The listing builds one solid part. Answer for the finished solid, in the listing's coordinates (mm). Face numbers are marked on the shaded views. A direction names the side the tool comes from. Coordinates: 2 decimals unless noted, no trailing zeros. Order: outer loops, then holes, each group sorted by start corner. A loop starts at its lowest first (then second) coordinate and runs counter-clockwise, first axis right, second up. Notation, with made-up numbers: (78, 56.25) -> (91, 56.25) arc R23 ccw to (91, 82.25) -> close; hole circle Ø1 at (88, 30). An arc over 180 degrees is marked (long way). Answer in a Markdown table with one row per item.
```python
from build123d import *

# Parameters (mm, degrees)
BOSS_EXTRU_1_DEPTH      = 17
ESQUISSE2_W             = 26
ESQUISSE2_H             = 16
BOSS_EXTRU_2_DEPTH      = 44
ENL_V_MAT_EXTRU_1_DEPTH = 12
ESQUISSE4_W             = 35
ESQUISSE4_H             = 16.981352254
BOSS_EXTRU_3_DEPTH      = 16
ESQUISSE5_W             = 35
ESQUISSE5_H             = 10
BOSS_EXTRU_4_DEPTH      = 44
ESQUISSE6_W             = 36.437850792
ESQUISSE6_H             = 10
BOSS_EXTRU_5_DEPTH      = 10
CONG_1_SIZE             = 10
CONG_1_SIZE_2           = 8
ESQUISSE8_R             = 5
ENL_V_MAT_EXTRU_2_DEPTH = 10


with BuildPart() as part:
    # Esquisse1 → Boss.-Extru.1 (new body)
    with BuildSketch(Plane.XY):
        Polygon((0, 0), (94, 0), (94, 9), (79, 16), (15, 16), (0, 9), align=None)
    extrude(amount=-BOSS_EXTRU_1_DEPTH)

    # Esquisse2 → Boss.-Extru.2 (add)
    with BuildSketch(Plane.XY):
        with Locations((47, 8)):
            Rectangle(ESQUISSE2_W, ESQUISSE2_H)
    extrude(amount=BOSS_EXTRU_2_DEPTH)

    # Esquisse3 → Enlèv. mat.-Extru.1 (cut)
    with BuildSketch(Plane(origin=(0, 16, 0), x_dir=(1, 0, 0), z_dir=(0, 1, 0))):
        with BuildLine():
            Line((38, -44), (56, -44))
            Line((56, -44), (56, -19))
            ThreePointArc((56, -19), (47, -10), (38, -19))
            Line((38, -19), (38, -44))
        make_face()
    extrude(amount=-ENL_V_MAT_EXTRU_1_DEPTH, mode=Mode.SUBTRACT)

    # Esquisse4 → Boss.-Extru.3 (add)
    with BuildSketch(Plane(origin=(0, 16, 0), x_dir=(1, 0, 0), z_dir=(0, 1, 0))):
        with Locations((47, 8.509323873)):
            Rectangle(ESQUISSE4_W, ESQUISSE4_H)
    extrude(amount=BOSS_EXTRU_3_DEPTH)

    # Esquisse5 → Boss.-Extru.4 (add)
    with BuildSketch(Plane(origin=(0, 0, -17), x_dir=(-1, 0, 0), z_dir=(0, 0, -1))):
        with Locations((-47, 27)):
            Rectangle(ESQUISSE5_W, ESQUISSE5_H)
    extrude(amount=BOSS_EXTRU_4_DEPTH)

    # Esquisse6 → Boss.-Extru.5 (add)
    with BuildSketch(Plane(origin=(0, 32, 0), x_dir=(1, 0, 0), z_dir=(0, 1, 0))):
        with Locations((46.281074604, 56)):
            Rectangle(ESQUISSE6_W, ESQUISSE6_H)
    extrude(amount=BOSS_EXTRU_5_DEPTH)

    # Congé1
    # an asymmetric fillet: 10, 8 mm, written as the material it takes off along each edge
    with BuildSketch(Plane(origin=(4.5, 32, -0.018647746), x_dir=(0, 0, -1), z_dir=(1, 0, 0))) as cong_1_piece_1:
        with BuildLine():
            Bezier((CONG_1_SIZE, 0), (0, 0), (0, -CONG_1_SIZE_2), weights=[1, 0.707106781, 1])
            Line((0, -CONG_1_SIZE_2), (0, 0))
            Line((0, 0), (CONG_1_SIZE, 0))
        make_face()
    extrude(amount=85, mode=Mode.SUBTRACT)

    # Esquisse8 → Enlèv. mat.-Extru.2 (cut)
    with BuildSketch(Plane(origin=(0, 32, 0), x_dir=(1, 0, 0), z_dir=(0, 1, 0))):
        with Locations(Location((47, 38.5, 0), (0, 0, 180))):
            Circle(ESQUISSE8_R)
    extrude(amount=-ENL_V_MAT_EXTRU_2_DEPTH, mode=Mode.SUBTRACT)

    # Esquisse9 → Lissage2 section 0
    with BuildSketch(Plane.XY.offset(-51)):
        with BuildLine():
            Line((41.281074604, 42), (51.281074604, 42))
            ThreePointArc((51.281074604, 42), (46.281074604, 47), (41.281074604, 42))
        make_face()
    # Esquisse10 → Lissage2 section 1
    with BuildSketch(Plane(origin=(0, 0, -61), x_dir=(-1, 0, 0), z_dir=(0, 0, -1))):
        with BuildLine():
            Line((-33.281074604, 42), (-59.281074604, 42))
            ThreePointArc((-59.281074604, 42), (-46.281074604, 55), (-33.281074604, 42))
        make_face()
    loft()


solid = part.part
```
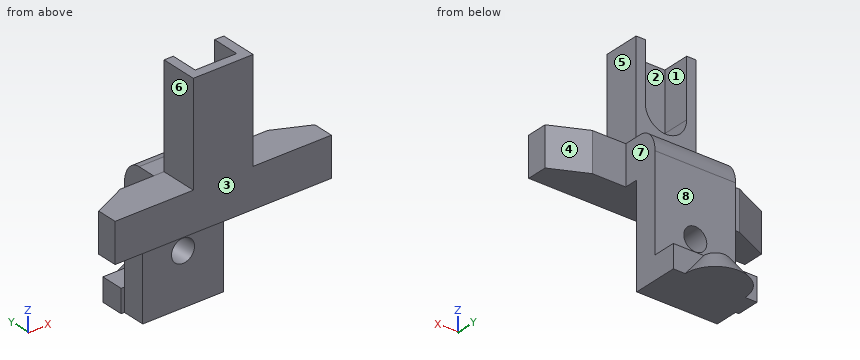
(1) A cutting plane is placed at D-D, the plane x = 22. Determine the outline of the cut face in (y, z).
Check values:
| item | result |
|---|---|
| outline | (0, -17) -> (16, -17) -> (16, 0) -> (0, 0) -> close |
(2) A cutting plane is placed at B-B, the plane y = 6.5. Determine the outline of the cut face in (x, z).
Check values:
| item | result |
|---|---|
| outline | (0, -17) -> (94, -17) -> (94, 0) -> (60, 0) -> (60, 44) -> (56, 44) -> (56, 19) arc R9 cw to (38, 19) -> (38, 44) -> (34, 44) -> (34, 0) -> (0, 0) -> close |
(3) A cutting plane is placed at C-C, the plane z = 4.5. Determine the outline of the cut face in (x, y), then the cut area to 3 significant figures.
Check values:
| item | result |
|---|---|
| outline | (34, 0) -> (60, 0) -> (60, 16) -> (34, 16) -> close |
| area | 416 mm² |
(4) A cutting plane is placed at A-A, the plane z = -38.5. Determine the outline of the cut face in (x, y), then the cut area to 3 significant figures.
Check values:
| item | result |
|---|---|
| outline | (29.5, 22) -> (42, 22) -> (42, 32) -> (29.5, 32) -> close; (52, 22) -> (64.5, 22) -> (64.5, 32) -> (52, 32) -> close |
| area | 250 mm² |
(5) Find the intervals of material crossed by line 1 along Y through (x, z) = (36, 39); line 2 along Z through (x, y) = (62, 23.5); line 3 along Z through (x, y) = (67, 6), in increasing order. Write a range as from..to.
Check values:
| item | result |
|---|---|
| line 1 | 0..16 |
| line 2 | -61..-0.02 |
| line 3 | -17..0 |
(6) Which of the six approach directions +Z, -Z, +X, -X, +Y, -Y give full straight-line access (tool end or side, diameter ignored) to the marked faces 5, 6, 7 and 8?
Check values:
| item | result |
|---|---|
| face 5 | +Z, +X, +Y, -Y |
| face 6 | +Z, -X, +Y, -Y |
| face 7 | +Z, -Z, +X, +Y |
| face 8 | +Z, +X, -X, +Y |
(7) Flat-ended cylindrical pins translate along their axes: pin 1 (8 mm diameter, centred on x = 58.5, z = -58.5, fed in from +Y); pin 2 (5 mm diameter, centred on x = 18, y = 11.5, fed in from +Z); pin 3 (12 mm diameter, centred on x = 34.5, z = 24, fed in from -Y); pin 4 (13 mm diameter, centred on y = 11.5, z = 28.5, fed in from -X). Find the tip coordinate at first contact, or state that the pin passes through.
Check values:
| item | result |
|---|---|
| pin 1 | y = 51.29 |
| pin 2 | z = 0 |
| pin 3 | y = 0 |
| pin 4 | x = 34 |
(8) For a pull along X with two mould halves and no side action, classify the marked faces 1, 2, 3 and 4 as released by +X, released by -X, zero draft, split by the parting line, or undercut.
Check values:
| item | result |
|---|---|
| face 1 | undercut |
| face 2 | undercut |
| face 3 | zero draft |
| face 4 | released by +X |
